Verification items for this drawing (mm, ordinates from the low corner). A direction names the side the tool comes from. Give positions to 0.01 mm unless a question says otherwise; leave off trailing zeros. Order: outer loops, then holes, each group sorted by start corner. A loop starts at its lowest first (then second) coordinate and runs counter-clockwise, first axis right, second up.
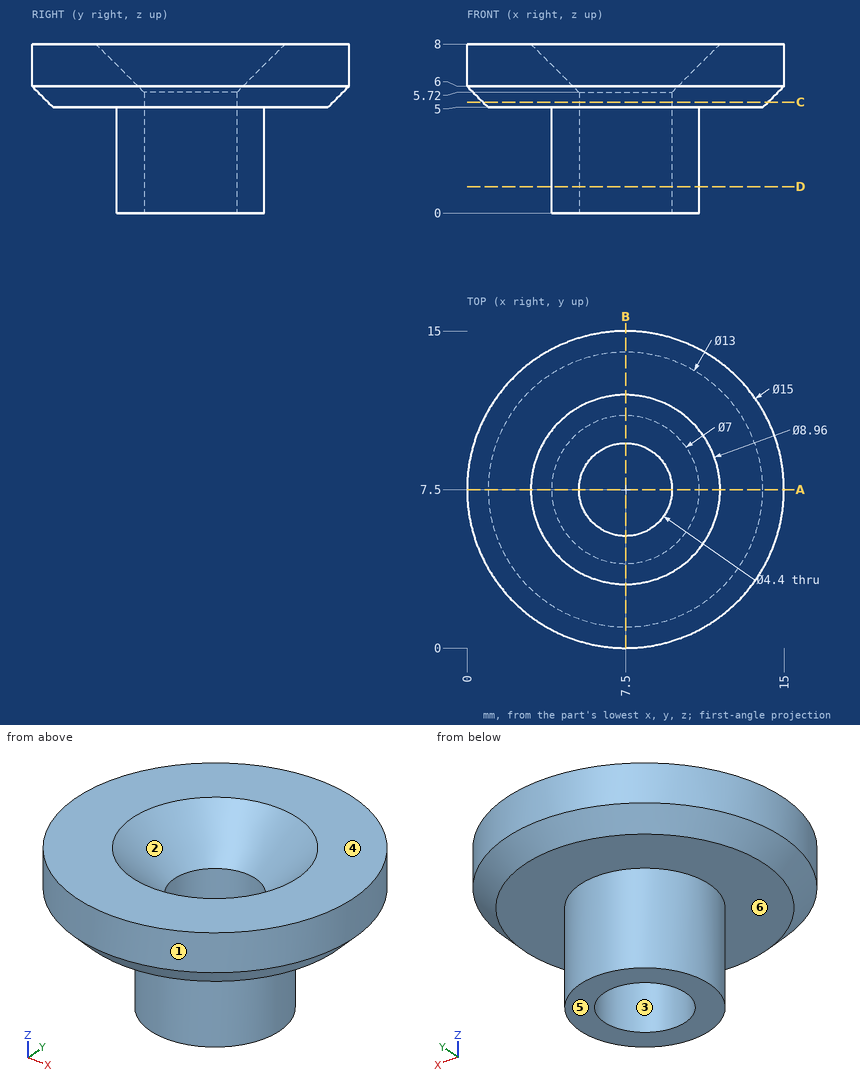
Q1. Cross-section at A-A, the plane y = 7.5. Record the boundary of the cut face in (x, z).
Q2. Access from +Z, -Z, +X, -X, +Y, -Y to the whole of each face (thin tool, end or side, straight path). Record for the marked faces 5 and 6.
Q3. Thickness scan on L1, parallel to Y at x = 7.5, z = 1.4; L2, parallel to X at y = 8, z = 2; L3, parallel to Y at x = 7.75, z = 6.75. Record the ranges inside material, lowest first.
Q4. Cross-section at D-D, the plane z = 1.25. Record the boundary of the cut face in (x, y).
Q5. Release check for a two-part mould opening along Y. For the marked faces 1, 2, 3 and 4 record: pulls with the +Y half, pulls with the -Y half, needs draft (parallel to the pull), parting line crosses it, or undercut.
Q6. Cross-section at C-C, the plane z = 5.25. Record the boundary of the cut face in (x, y), and give its area (3 significant figures).
Q7. Gauge pin test, flat ends, axial feed: P1, Ø2, axis at x = 3, z = 5, coming from the -Y side; P2, Ø3, axis at y = 9, z = 1.5, coming from the -X side; P3, Ø3.5, axis at x = 7.5, y = 7.5, coming from the +Z side; P4, Ø3, axis at x = 5, y = 9, coming from the +Z side. Record the tip position at first contact, or that the pin passes through.
Answers follow:
1. outline: (0, 6) - (1, 5) - (4, 5) - (4, 0) - (5.3, 0) - (5.3, 5.72) - (3.02, 8) - (0, 8) - close; (9.7, 0) - (11, 0) - (11, 5) - (14, 5) - (15, 6) - (15, 8) - (11.98, 8) - (9.7, 5.72) - close
2. face 5: -Z, +X, -X, +Y, -Y
2. face 6: -Z
3. L1: y = 4 to 5.3, 9.7 to 11
3. L2: x = 4.04 to 5.36, 9.64 to 10.96
3. L3: y = 0 to 4.28, 10.72 to 15
4. outline: circle Ø7 at (7.5, 7.5); hole circle Ø4.4 at (7.5, 7.5)
5. face 1: parting line crosses it
5. face 2: undercut
5. face 3: undercut
5. face 4: needs draft
6. outline: circle Ø13.5 at (7.5, 7.5); hole circle Ø4.4 at (7.5, 7.5)
6. area: 128 mm2
7. P1: stops at y = 1.31
7. P2: stops at x = 4
7. P3: passes through
7. P4: stops at z = 7.94
